The drawing under review shows one solid part. Ordinate dimensions are in mm from its lowest x, y, z. A direction names the side the tool comes from. Give positions to 0.01 mm unless a question says otherwise; leave off trailing zeros. Write each loop counter-clockwise with the first axis right and the second up, starting at its lowest first coordinate (ties: lowest second). Pieces come first, ordered by that corner, then holes.
Q1. We need section A-A (y = 14). Write out the cut boundary in (x, z), then the cut area to 3 significant figures.
Q2. Machinability: for the marked faces 1 and 2, which of the approach directions +Z, -Z, +X, -X, +Y, -Y give a long, thin tool a straight path to every point of the face, cutting with its end or side? Answer none if there is none.
Q3. We need section B-B (x = 14). Write out the cut boundary in (y, z).
Q4. We need section C-C (z = 29). Write out the cut boundary in (x, y), then the cut area to 3 significant figures.
Q5. We need section D-D (z = 7). Write out the cut boundary in (x, y).
Q6. For line 1 (Z direction, x = 24.5, y = 20); line 2 (Y direction, x = 7.5, z = 37); line 3 (X direction, y = 6, z = 37), list the stretches that pass through material, from the lowest coordinate up.
Q7. Insertion check: P1, Ø5, axis at x = 8, y = 17.5, coming from the -Z side; P2, Ø10, axis at x = 7, z = 11, coming from the +Y side; P3, Ø0.9, axis at y = 28.5, z = 25, coming from the +X side. Each pin has a flat end and moves straight along its axis. Give the tip position at first contact, or say it passes through.
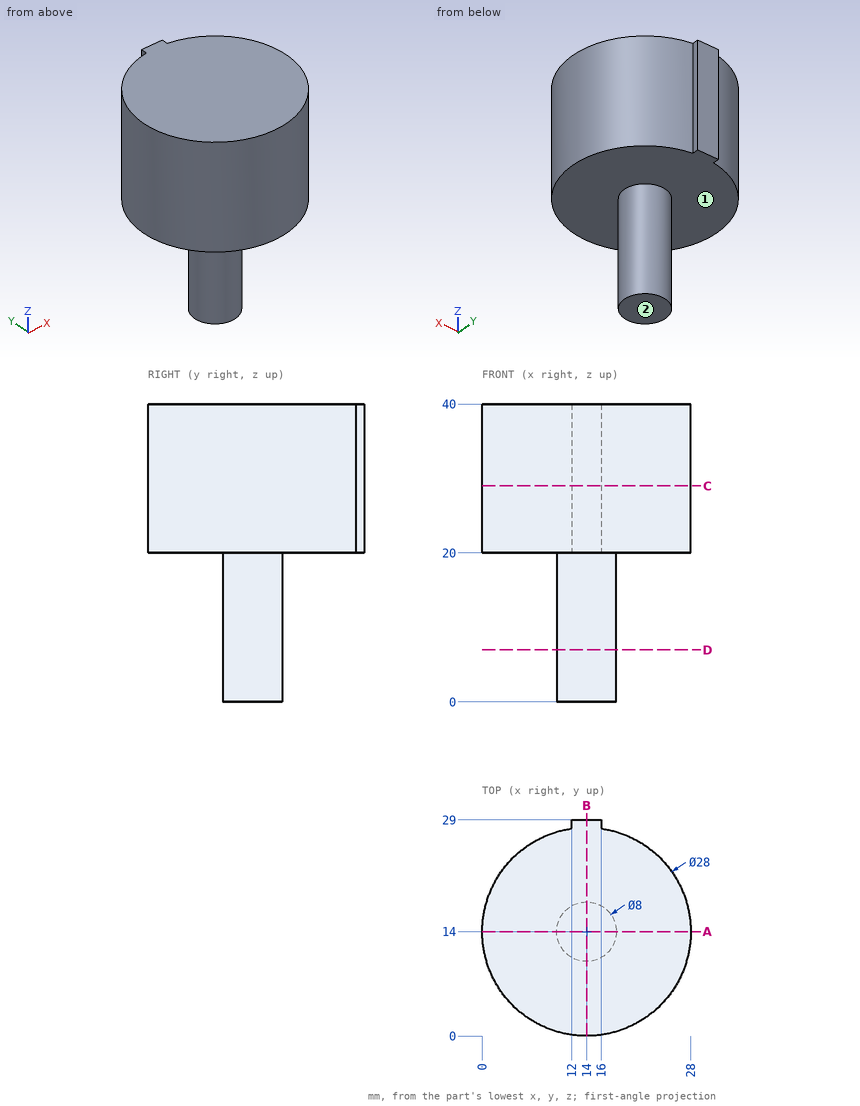
Computed:
1. outline: (0, 20) - (10, 20) - (10, 0) - (18, 0) - (18, 20) - (28, 20) - (28, 40) - (0, 40) - close
1. area: 720 mm2
2. face 1: -Z
2. face 2: -Z, +X, -X, +Y, -Y
3. outline: (0, 20) - (10, 20) - (10, 0) - (18, 0) - (18, 20) - (29, 20) - (29, 40) - (0, 40) - close
4. outline: (12, 27.86) arc R14 ccw (long way) to (16, 27.86) - (16, 29) - (12, 29) - close
4. area: 620 mm2
5. outline: circle Ø8 at (14, 14)
6. line 1: z = 20 to 40
6. line 2: y = 1.6 to 26.4
6. line 3: x = 2.51 to 25.49
7. P1: stops at z = 20
7. P2: stops at y = 17.46
7. P3: stops at x = 16
